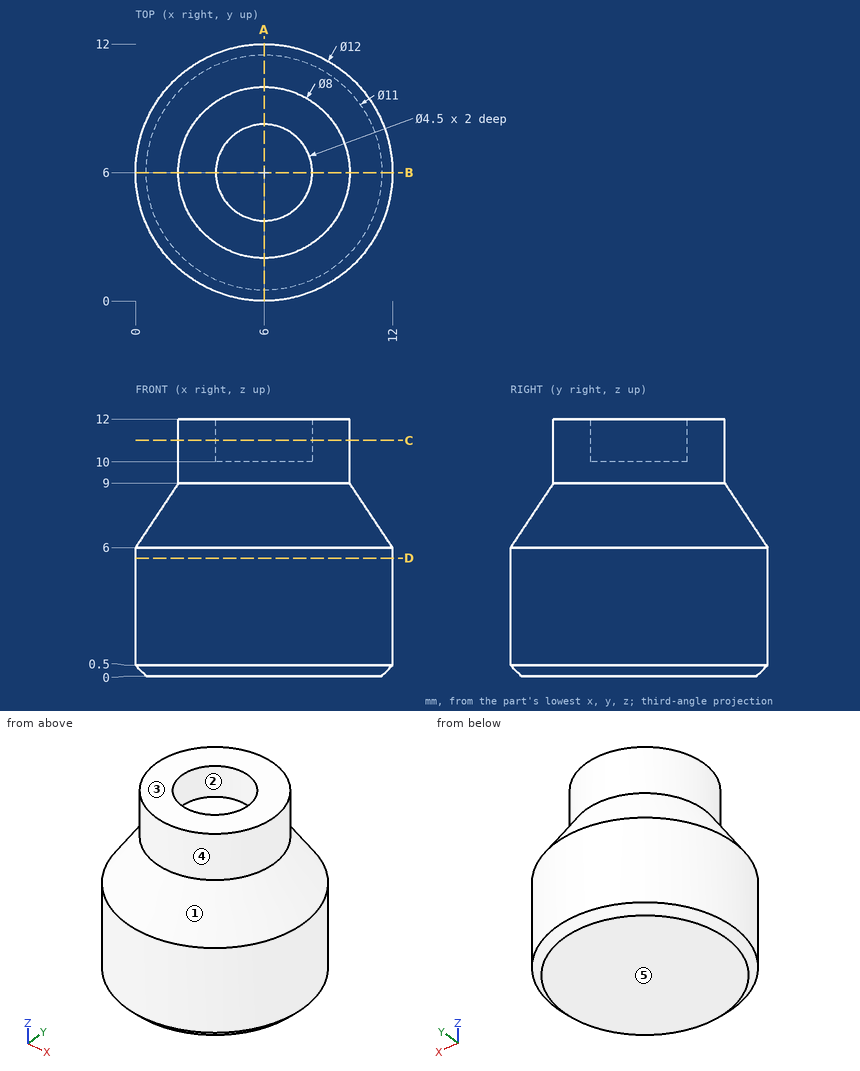
The figure shows three views and two pictorial views of one solid part (mm, origin at its lowest corner). Answer the questions. A direction names the side the tool comes from. Give positions to 0.01 mm unless a question says otherwise; leave off trailing zeros. Loops run counter-clockwise (first coordinate to the right, second up) from the corner with the lowest first, then second, coordinate; pieces in that order, holes last. Notation, with made-up numbers: (67.5, 49) -> (82.5, 49) arc R9 ccw to (82.5, 61) -> close; hole circle Ø8 at (-19, -3.75). An arc over 180 degrees is marked (long way). Use CSV: the item, a comma, the result in double quotes.
1. Straight lines are drawn through the part: line 1 (Y direction, x = 6, z = 10.45); line 2 (Z direction, x = 6.75, y = 8); line 3 (Z direction, x = 6, y = 1.5). For each, find the intervals that lie inside material, in ascending order.
Found:
line 1,"2 to 3.75, 8.25 to 10"
line 2,"0 to 10"
line 3,"0 to 8.25"
2. The mould has two halves that part along X. Classify the marked faces 1, 2 and 3: +X half, -X half, draft (parallel to the pull), parting line (faces both ways), or undercut.
Found:
face 1,"parting line"
face 2,"undercut"
face 3,"draft"
3. The part is cut by section D-D (z = 5.5). Write down the section's boundary in (x, y), then the cut area to 3 significant figures.
Found:
outline,"circle Ø12 at (6, 6)"
area,"113 mm^2"
4. Flat-ended cylindrical pins translate along their axes: pin 1 Ø1 at (y, z) = (1.5, 2.5) entering from -X; pin 2 Ø5 at (x, z) = (9, 10.5) entering from +Y; pin 3 Ø1 at (x, z) = (10.5, 1.5) entering from -Y; pin 4 Ø4 at (x, y) = (3, 5.5) entering from -Z. Find the tip coordinate at first contact, or state that the pin passes through.
Found:
pin 1,"x = 1.53"
pin 2,"y = 10.08"
pin 3,"y = 1.53"
pin 4,"z = 0"
5. A tool of negligible diameter and unlimited length cuts with its end or side. For the marked faces 4 and 5, from which of +Z, -Z, +X, -X, +Y, -Y can it reach the whole face along a straight path? Write none if from no direction.
Found:
face 4,"+Z"
face 5,"-Z, +X, -X, +Y, -Y"
6. The part is cut by section C-C (z = 11). Write down the section's boundary in (x, y), then the cut area to 3 significant figures.
Found:
outline,"circle Ø8 at (6, 6); hole circle Ø4.5 at (6, 6)"
area,"34.4 mm^2"
7. The part is cut by section A-A (x = 6). Write down the section's boundary in (y, z), then the cut area to 3 significant figures.
Found:
outline,"(0, 0.5) -> (0.5, 0) -> (11.5, 0) -> (12, 0.5) -> (12, 6) -> (10, 9) -> (10, 12) -> (8.25, 12) -> (8.25, 10) -> (3.75, 10) -> (3.75, 12) -> (2, 12) -> (2, 9) -> (0, 6) -> close"
area,"117 mm^2"
